Check sheet for the modelled part. Datum: model origin and axes. Units: mm. Coordinates: 2 decimals unless noted, no trailing zeros. Order: outer loops, then holes, each group sorted by start corner. A loop starts at its lowest first (then second) coordinate and runs counter-clockwise, first axis right, second up.
from build123d import *

# Parameters (mm, degrees)
SKETCH1_W             = 15.8
SKETCH1_H             = 15.8
BASE_DEPTH            = 3.2
BOTTOM_CUT_DEPTH      = 2
SKETCH3_R             = 4
SKETCH3_R_2           = 2.4
LAMP_POST_DEPTH       = 128
WIRE_BOTTOM_CUT_REACH = 5.2
SKETCH4_R             = 2.4


with BuildPart() as part:
    # Sketch1 → Base (new body)
    with BuildSketch(Plane(origin=(0, 0, 0), x_dir=(1, 0, 0), z_dir=(0, 1, 0))):
        Rectangle(SKETCH1_W, SKETCH1_H)
    extrude(amount=BASE_DEPTH)

    # Sketch2 → Bottom cut (cut)
    with BuildSketch(Plane.XZ):
        with BuildLine():
            Line((6.6, -6.6), (6.6, 6.6))
            Line((6.6, 6.6), (-6.6, 6.6))
            Line((-6.6, 6.6), (-6.6, -6.6))
            Line((-6.6, -6.6), (-1.25, -6.6))
            Line((-1.25, -6.6), (-1.25, -3.161882351))
            ThreePointArc((-1.25, -3.161882351), (-1.911805429, 2.811583184), (3.4, 0))
            ThreePointArc((3.4, 0), (2.811583184, -1.911805429), (1.25, -3.161882351))
            Line((1.25, -3.161882351), (1.25, -6.6))
            Line((1.25, -6.6), (6.6, -6.6))
        make_face()
        with BuildLine():
            ThreePointArc((-1.25, -2.165063509), (0, -2.5), (1.25, -2.165063509))
            Line((1.25, -2.165063509), (-1.25, -2.165063509))
        make_face()
        with BuildLine():
            Line((-1.25, -2.165063509), (1.25, -2.165063509))
            ThreePointArc((1.25, -2.165063509), (2.165063509, -1.25), (2.5, 0))
            ThreePointArc((2.5, 0), (-1.25, 2.165063509), (-1.25, -2.165063509))
        make_face()
        with BuildLine():
            Line((-1.25, -6.6), (1.25, -6.6))
            Line((1.25, -6.6), (1.25, -3.161882351))
            ThreePointArc((1.25, -3.161882351), (0, -3.4), (-1.25, -3.161882351))
            Line((-1.25, -3.161882351), (-1.25, -6.6))
        make_face()
    extrude(amount=-BOTTOM_CUT_DEPTH, mode=Mode.SUBTRACT)

    # Sketch3 → Lamp post (add)
    with BuildSketch(Plane(origin=(0, 3.2, 0), x_dir=(1, 0, 0), z_dir=(0, 1, 0))):
        Circle(SKETCH3_R)
        Circle(SKETCH3_R_2, mode=Mode.SUBTRACT)
    extrude(amount=LAMP_POST_DEPTH)

    # Sketch4 → Wire bottom cut (cut, up to next)
    with BuildSketch(Plane(origin=(0, 3.2, 0), x_dir=(1, 0, 0), z_dir=(0, 1, 0)), mode=Mode.PRIVATE) as wire_bottom_cut_sk1:
        Circle(SKETCH4_R)
    wire_bottom_cut_tool1 = extrude(wire_bottom_cut_sk1.sketch, amount=-WIRE_BOTTOM_CUT_REACH, mode=Mode.PRIVATE) & part.part
    add(wire_bottom_cut_tool1.solids().sort_by_distance((0, 3.2, 0))[0], mode=Mode.SUBTRACT)


solid = part.part
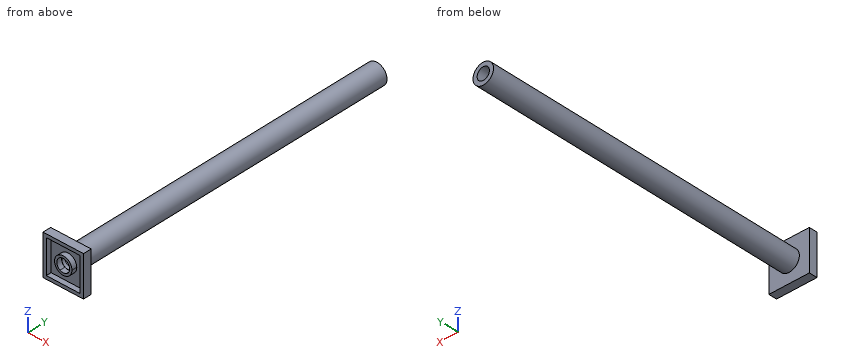
(1) Thickness scan on probe 1 along X at (y, z) = (92, 0); probe 2 along X at (y, z) = (2.6, 0). Record the ranges inside material, lowest first.
Filled in:
probe 1: x = -4 to -2.4, 2.4 to 4
probe 2: x = -7.9 to -2.4, 2.4 to 7.9
(2) Go/stop test with flat-tipped pins: P1, Ø6, axis at x = 3, y = 40, coming from the -Z side; P2, Ø4, axis at y = 93, z = -5, coming from the -X side; P3, Ø4, axis at x = -2.5, y = 108.5, coming from the +Z side. Record where each tip stops, or that it passes through.
Filled in:
P1: stops at z = -4
P2: stops at x = -2.65
P3: stops at z = 3.97
(3) Cross-section at B-B (y = 79.5). Enter the section's corners in (x, z), and give its area (3 significant figures).
Filled in:
outline: circle Ø8 at (0, 0); hole circle Ø4.8 at (0, 0)
area: 32.2 mm2
(4) Cross-section at A-A (x = 0). Enter the section's corners in (y, z), and give its area (3 significant figures).
Filled in:
outline: (0, -7.9) - (3.2, -7.9) - (3.2, -4) - (131.2, -4) - (131.2, -2.4) - (2, -2.4) - (2, -2.5) - (0, -2.5) - (0, -3.4) - (2, -3.4) - (2, -6.6) - (0, -6.6) - close; (0, 2.5) - (2, 2.5) - (2, 2.4) - (131.2, 2.4) - (131.2, 4) - (3.2, 4) - (3.2, 7.9) - (0, 7.9) - (0, 6.6) - (2, 6.6) - (2, 3.4) - (0, 3.4) - close
area: 432 mm2
